Source: CAD feature listing. Evaluate the final solid. Frame: model axes, mm. A direction names the side the tool comes from. Coordinates: 2 decimals unless noted, no trailing zeros. Order: outer loops, then holes, each group sorted by start corner. A loop starts at its lowest first (then second) coordinate and runs counter-clockwise, first axis right, second up.
```python
from build123d import *

# Parameters (mm, degrees)
SKETCH1_R           = 24.15
SKETCH1_R_2         = 21.15
BOSS_EXTRUDE1_DEPTH = 400


with BuildPart() as part:
    # Sketch1 → Boss-Extrude1 (new body)
    with BuildSketch(Plane(origin=(0, 0, 0), x_dir=(0, 0, -1), z_dir=(1, 0, 0))):
        Circle(SKETCH1_R)
        Circle(SKETCH1_R_2, mode=Mode.SUBTRACT)
    extrude(amount=-BOSS_EXTRUDE1_DEPTH)

    # Sketch2 → Cut-Revolve1 (revolve, cut)
    with BuildSketch(Plane.XY):
        Polygon((0, 24.15), (-30, 24.15), (0, 23.495397671), align=None)
    revolve(axis=Axis((0, 0, 0), (1, 0, 0)), mode=Mode.SUBTRACT)

    # Sketch3 → Cut-Revolve2 (revolve, cut)
    with BuildSketch(Plane.XY):
        Polygon((-400, 24.15), (-370, 24.15), (-400, 23.495397671), align=None)
    revolve(axis=Axis((-400, 0, 0), (1, 0, 0)), mode=Mode.SUBTRACT)


solid = part.part
```
Q1. Section query C-C on x = -189. Output: boundary loops of the cut face in (y, z).
Solutions:
outline: circle Ø48.3 at (0, 0); hole circle Ø42.3 at (0, 0)
Q2. Pull-direction query (Z, two-part tool) for faces 1 (the cylindrical face through (-197.2, -20.65, 4.58)), 2 (the cylindrical face through (-197.62, 7.254, -23.035)), 3 (the flat face through (-400, 4, 21)); classes: pulls with the +Z half, pulls with the -Z half, needs draft (parallel to the pull), parting line crosses it, or undercut.
Solutions:
face 1: undercut
face 2: parting line crosses it
face 3: needs draft
Q3. Set-up query: faces 4 (the conical face through (-385.21, 22.72, 7.15)), 5 (the conical face through (-14.79, 22.72, 7.15)), 6 (the flat face through (0, 4, 21)). Return all of +Z, -Z, +X, -X, +Y, -Y with unobstructed straight access to the full face (end or side cutting, diameter ignored); none if empty.
Solutions:
face 4: -X
face 5: +X
face 6: +Z, -Z, +X, +Y, -Y
Q4. Section query A-A on y = 0. Output: boundary loops of the cut face in (x, z), plus the area to 3 significant figures.
Solutions:
outline: (-400, -23.5) - (-370, -24.15) - (-30, -24.15) - (0, -23.5) - (0, -21.15) - (-400, -21.15) - close; (-400, 21.15) - (0, 21.15) - (0, 23.5) - (-30, 24.15) - (-370, 24.15) - (-400, 23.5) - close
area: 2,360 mm2
Q5. Material intervals for line 1 along Y through (x, z) = (-192, 0); line 2 along Y through (x, z) = (-376, -2.5); line 3 along Z through (x, y) = (-62, -13.5), sorted ascending.
Solutions:
line 1: y = -24.15 to -21.15, 21.15 to 24.15
line 2: y = -23.89 to -21, 21 to 23.89
line 3: z = -20.02 to -16.28, 16.28 to 20.02
Q6. Pin query (flat end, axial travel): P1, Ø5, axis at x = -306.5, z = 14, coming from the -Y side; P2, Ø6, axis at x = -298, z = 12.5, coming from the +Y side; P3, Ø10, axis at x = -93.5, y = -14, coming from the +Z side. Return the tip coordinate at first contact, or that it passes through.
Solutions:
P1: stops at y = -21.24
P2: stops at y = 22.2
P3: stops at z = 22.41
